from build123d import *

# Parameters (mm, degrees)
SKETCH1_R           = 16.515
BOSS_EXTRUDE1_DEPTH = 19
SKETCH2_R           = 3.5
CUT_EXTRUDE1_DEPTH  = 17.515
SKETCH4_R           = 1
CUT_EXTRUDE2_DEPTH  = 19


with BuildPart() as part:
    # Sketch1 → Boss-Extrude1 (new body)
    with BuildSketch(Plane.XY):
        Circle(SKETCH1_R)
    extrude(amount=BOSS_EXTRUDE1_DEPTH)

    # Sketch2 → Cut-Extrude1 (cut, through all)
    with BuildSketch(Plane(origin=(0, 0, 0), x_dir=(1, 0, 0), z_dir=(0, 1, 0))):
        with Locations((0, -9.045224282)):
            Circle(SKETCH2_R)
    extrude(amount=CUT_EXTRUDE1_DEPTH, mode=Mode.SUBTRACT)

    # Sketch4 → Cut-Extrude2 (cut)
    with BuildSketch(Plane(origin=(-17.320508076, 10, 0), x_dir=(0, 0, 1), z_dir=(-0.866025404, 0.5, 0))):
        with Locations((9.5, 0)):
            Circle(SKETCH4_R)
    extrude(amount=-CUT_EXTRUDE2_DEPTH, mode=Mode.SUBTRACT)


solid = part.part
For this review, take the finished solid that the model builds, in its own axes (mm). A direction names the side the tool comes from. Round coordinates to 2 decimals unless told otherwise and drop trailing zeros. Order: outer loops, then holes, each group sorted by start corner. A loop starts at its lowest first (then second) coordinate and runs counter-clockwise, first axis right, second up. Notation, with made-up numbers: M -16,71.25 L 39,71.25 A24 ccw 39,103.25 Z; hole C 77.5,42 d5. An arc over 180 degrees is marked long. Write each question's results on one line, items separated by ' | '. Start each with the question number.
1. Add section A-A (x = 0). State the section outline as (y, z) points (3 decimals).
2. Add section C-C (z = 11). State the section outline as (x, y) points (3 decimals).
3. Draft analysis for pull direction Y (two halves, no side actions). For faces 1 (the face through (-1.658, -0.198, 9.487)), 2 (the face through (-9.19, 4.18, 9.28)), 3 (the face through (0, 0, 0)), state which applies: pulls with the +Y half, pulls with the -Y half, needs draft (parallel to the pull), parting line crosses it, or undercut.
4. To check wall thickness, follow L1, parallel to Z at x = 0, y = 5; L2, parallel to X at y = 14, z = 6; L3, parallel to X at y = 14, z = 6.5. State the ranges of each line that lie inside material, in increasing order. Write a range as [from, to].
5. Clearance check with flat-ended pins moving along their axes: pin 1 Ø1 at (x, z) = (3, 17) entering from +Y; pin 2 Ø6 at (x, z) = (7, 8) entering from -Y. State where each tip first meets the part, or that it passes through.
6. Add section D-D (x = 13). State the section outline as (y, z) points, then the cut area to 3 significant figures.
7. Add section B-B (y = 11). State the section outline as (x, z) points.
8. Tool access review of faces 4 (the face through (0, 0, 9)), 5 (the face through (0, 0, 19)): name each direction out of +Z, -Z, +X, -X, +Y, -Y from which nothing blocks a thin tool from reaching the whole face with its end or side.
Output values:
1) outline: M -16.515,0 L 16.515,0 L 16.515,5.545 L 0,5.545 L 0,12.545 L 16.515,12.545 L 16.515,19 L -16.515,19 Z
2) outline: M -2.903,0 L -2.903,16.258 A16.515 ccw long 2.903,16.258 L 2.903,0 Z
3) face 1: pulls with the +Y half | face 2: undercut | face 3: needs draft
4) L1: [0, 5.55], [12.55, 19] | L2: [-8.76, -1.73], [1.73, 8.76] | L3: [-8.76, -2.4], [2.4, 8.76]
5) pin 1: y = 16.32 | pin 2: y = -16.02
6) outline: M -10.19,0 L 10.19,0 L 10.19,19 L -10.19,19 Z | area: 387 mm^2
7) outline: M -12.32,0 L 12.32,0 L 12.32,19 L -12.32,19 Z; hole C 0,9.05 d7
8) face 4: +Y | face 5: +Z, +X, -X, +Y, -Y
